Design review of the part built by this model. Coordinates are the model's own, in mm. A direction names the side the tool comes from. Give positions to 0.01 mm unless a question says otherwise; leave off trailing zeros. Loops run counter-clockwise (first coordinate to the right, second up) from the corner with the lowest first, then second, coordinate; pieces in that order, holes last. Notation, with made-up numbers: (3, 6.5) -> (53, 6.5) arc R17 ccw to (53, 36.5) -> close; hole circle Ø8 at (82, 65.5). An arc over 180 degrees is marked (long way). Answer as CSV lines item,"result".
from build123d import *

# Parameters (mm, degrees)
SKETCH1_W            = 122
SKETCH1_H            = 88
BOSS_EXTRUDE1_DEPTH  = 54
BOSS_EXTRUDE2_START  = -1
SKETCH2_W            = 118
SKETCH2_H            = 84
BOSS_EXTRUDE2_DEPTH  = 53
BOSS_EXTRUDE3_START  = 50
SKETCH3_W            = 97
SKETCH3_H            = 56
BOSS_EXTRUDE3_DEPTH  = 10
BOSS_EXTRUDE4_START  = 50
SKETCH4_R            = 4.5
BOSS_EXTRUDE4_DEPTH  = 10
BOSS_EXTRUDE5_START  = 50
SKETCH5_W            = 12
SKETCH5_H            = 6
BOSS_EXTRUDE5_DEPTH  = 10
BOSS_EXTRUDE6_START  = -65
SKETCH6_R            = 1.2
BOSS_EXTRUDE6_DEPTH  = 130
BOSS_EXTRUDE7_START  = 55
SKETCH7_R            = 1.5
BOSS_EXTRUDE7_DEPTH  = 10
BOSS_EXTRUDE8_START  = 55
SKETCH8_R            = 1.5
BOSS_EXTRUDE8_DEPTH  = 10
BOSS_EXTRUDE9_START  = 55
SKETCH9_R            = 1.5
BOSS_EXTRUDE9_DEPTH  = 10
BOSS_EXTRUDE10_START = 55
SKETCH10_R           = 1.5
BOSS_EXTRUDE10_DEPTH = 10
BOSS_EXTRUDE11_START = 55
SKETCH11_R           = 1.5
BOSS_EXTRUDE11_DEPTH = 10
BOSS_EXTRUDE12_START = 55
SKETCH12_R           = 1.5
BOSS_EXTRUDE12_DEPTH = 10
BOSS_EXTRUDE13_START = 55
SKETCH13_R           = 1.5
BOSS_EXTRUDE13_DEPTH = 10
BOSS_EXTRUDE14_START = 55
SKETCH14_R           = 1.5
BOSS_EXTRUDE14_DEPTH = 10
BOSS_EXTRUDE15_START = 55
SKETCH15_R           = 1.5
BOSS_EXTRUDE15_DEPTH = 10
BOSS_EXTRUDE16_START = 12
SKETCH16_W           = 30
SKETCH16_H           = 4
BOSS_EXTRUDE16_DEPTH = 30
BOSS_EXTRUDE17_START = -65
SKETCH17_R           = 1.1
BOSS_EXTRUDE17_DEPTH = 130
BOSS_EXTRUDE18_START = -65
SKETCH18_R           = 1.1
BOSS_EXTRUDE18_DEPTH = 130


with BuildPart() as part:
    # Sketch1 → Boss-Extrude1 (new body)
    with BuildSketch(Plane.XY):
        with Locations((0, 44)):
            Rectangle(SKETCH1_W, SKETCH1_H)
    extrude(amount=BOSS_EXTRUDE1_DEPTH)


with BuildPart() as body_2:
    # Sketch2 → Boss-Extrude2 (new body)
    with BuildSketch(Plane.XY.offset(BOSS_EXTRUDE2_START)):
        with Locations((0, 44)):
            Rectangle(SKETCH2_W, SKETCH2_H)
    extrude(amount=BOSS_EXTRUDE2_DEPTH)


with BuildPart() as part_1:
    add(part.part)

    # Combine1: cut body 2
    add(body_2.part, mode=Mode.SUBTRACT)


with BuildPart() as body_2_2:
    # Sketch3 → Boss-Extrude3 (new body)
    with BuildSketch(Plane.XY.offset(BOSS_EXTRUDE3_START)):
        with Locations((0, 42)):
            Rectangle(SKETCH3_W, SKETCH3_H)
    extrude(amount=BOSS_EXTRUDE3_DEPTH)


with BuildPart() as part_2:
    add(part_1.part)

    # Combine2: cut body 2 2
    add(body_2_2.part, mode=Mode.SUBTRACT)


with BuildPart() as body_2_3:
    # Sketch4 → Boss-Extrude4 (new body)
    with BuildSketch(Plane.XY.offset(BOSS_EXTRUDE4_START)):
        with Locations((0, 79)):
            Circle(SKETCH4_R)
    extrude(amount=BOSS_EXTRUDE4_DEPTH)


with BuildPart() as part_3:
    add(part_2.part)

    # Combine3: cut body 2 3
    add(body_2_3.part, mode=Mode.SUBTRACT)


with BuildPart() as body_2_4:
    # Sketch5 → Boss-Extrude5 (new body)
    with BuildSketch(Plane.XY.offset(BOSS_EXTRUDE5_START)):
        with Locations((34, 79)):
            Rectangle(SKETCH5_W, SKETCH5_H)
    extrude(amount=BOSS_EXTRUDE5_DEPTH)


with BuildPart() as part_4:
    add(part_3.part)

    # Combine4: cut body 2 4
    add(body_2_4.part, mode=Mode.SUBTRACT)


with BuildPart() as body_2_5:
    # Sketch6 → Boss-Extrude6 (new body)
    with BuildSketch(Plane(origin=(0, 0, 0), x_dir=(0, 0, -1), z_dir=(1, 0, 0)).offset(BOSS_EXTRUDE6_START)):
        with Locations((-27, 52)):
            Circle(SKETCH6_R)
    extrude(amount=BOSS_EXTRUDE6_DEPTH)


with BuildPart() as part_5:
    add(part_4.part)

    # Combine5: cut body 2 5
    add(body_2_5.part, mode=Mode.SUBTRACT)


with BuildPart() as body_2_6:
    # Sketch7 → Boss-Extrude7 (new body)
    with BuildSketch(Plane(origin=(0, 0, 0), x_dir=(0, 0, -1), z_dir=(1, 0, 0)).offset(BOSS_EXTRUDE7_START)):
        with Locations((-16, 20)):
            Circle(SKETCH7_R)
    extrude(amount=BOSS_EXTRUDE7_DEPTH)


with BuildPart() as part_6:
    add(part_5.part)

    # Combine6: cut body 2 6
    add(body_2_6.part, mode=Mode.SUBTRACT)


with BuildPart() as body_2_7:
    # Sketch8 → Boss-Extrude8 (new body)
    with BuildSketch(Plane(origin=(0, 0, 0), x_dir=(0, 0, -1), z_dir=(1, 0, 0)).offset(BOSS_EXTRUDE8_START)):
        with Locations((-24, 20)):
            Circle(SKETCH8_R)
    extrude(amount=BOSS_EXTRUDE8_DEPTH)


with BuildPart() as part_7:
    add(part_6.part)

    # Combine7: cut body 2 7
    add(body_2_7.part, mode=Mode.SUBTRACT)


with BuildPart() as body_2_8:
    # Sketch9 → Boss-Extrude9 (new body)
    with BuildSketch(Plane(origin=(0, 0, 0), x_dir=(0, 0, -1), z_dir=(1, 0, 0)).offset(BOSS_EXTRUDE9_START)):
        with Locations((-32, 20)):
            Circle(SKETCH9_R)
    extrude(amount=BOSS_EXTRUDE9_DEPTH)


with BuildPart() as part_8:
    add(part_7.part)

    # Combine8: cut body 2 8
    add(body_2_8.part, mode=Mode.SUBTRACT)


with BuildPart() as body_2_9:
    # Sketch10 → Boss-Extrude10 (new body)
    with BuildSketch(Plane(origin=(0, 0, 0), x_dir=(0, 0, -1), z_dir=(1, 0, 0)).offset(BOSS_EXTRUDE10_START)):
        with Locations((-16, 28)):
            Circle(SKETCH10_R)
    extrude(amount=BOSS_EXTRUDE10_DEPTH)


with BuildPart() as part_9:
    add(part_8.part)

    # Combine9: cut body 2 9
    add(body_2_9.part, mode=Mode.SUBTRACT)


with BuildPart() as body_2_10:
    # Sketch11 → Boss-Extrude11 (new body)
    with BuildSketch(Plane(origin=(0, 0, 0), x_dir=(0, 0, -1), z_dir=(1, 0, 0)).offset(BOSS_EXTRUDE11_START)):
        with Locations((-24, 28)):
            Circle(SKETCH11_R)
    extrude(amount=BOSS_EXTRUDE11_DEPTH)


with BuildPart() as part_10:
    add(part_9.part)

    # Combine10: cut body 2 10
    add(body_2_10.part, mode=Mode.SUBTRACT)


with BuildPart() as body_2_11:
    # Sketch12 → Boss-Extrude12 (new body)
    with BuildSketch(Plane(origin=(0, 0, 0), x_dir=(0, 0, -1), z_dir=(1, 0, 0)).offset(BOSS_EXTRUDE12_START)):
        with Locations((-32, 28)):
            Circle(SKETCH12_R)
    extrude(amount=BOSS_EXTRUDE12_DEPTH)


with BuildPart() as part_11:
    add(part_10.part)

    # Combine11: cut body 2 11
    add(body_2_11.part, mode=Mode.SUBTRACT)


with BuildPart() as body_2_12:
    # Sketch13 → Boss-Extrude13 (new body)
    with BuildSketch(Plane(origin=(0, 0, 0), x_dir=(0, 0, -1), z_dir=(1, 0, 0)).offset(BOSS_EXTRUDE13_START)):
        with Locations((-16, 36)):
            Circle(SKETCH13_R)
    extrude(amount=BOSS_EXTRUDE13_DEPTH)


with BuildPart() as part_12:
    add(part_11.part)

    # Combine12: cut body 2 12
    add(body_2_12.part, mode=Mode.SUBTRACT)


with BuildPart() as body_2_13:
    # Sketch14 → Boss-Extrude14 (new body)
    with BuildSketch(Plane(origin=(0, 0, 0), x_dir=(0, 0, -1), z_dir=(1, 0, 0)).offset(BOSS_EXTRUDE14_START)):
        with Locations((-24, 36)):
            Circle(SKETCH14_R)
    extrude(amount=BOSS_EXTRUDE14_DEPTH)


with BuildPart() as part_13:
    add(part_12.part)

    # Combine13: cut body 2 13
    add(body_2_13.part, mode=Mode.SUBTRACT)


with BuildPart() as body_2_14:
    # Sketch15 → Boss-Extrude15 (new body)
    with BuildSketch(Plane(origin=(0, 0, 0), x_dir=(0, 0, -1), z_dir=(1, 0, 0)).offset(BOSS_EXTRUDE15_START)):
        with Locations((-32, 36)):
            Circle(SKETCH15_R)
    extrude(amount=BOSS_EXTRUDE15_DEPTH)


with BuildPart() as part_14:
    add(part_13.part)

    # Combine14: cut body 2 14
    add(body_2_14.part, mode=Mode.SUBTRACT)


with BuildPart() as body_2_15:
    # Sketch16 → Boss-Extrude16 (new body)
    with BuildSketch(Plane.XY.offset(BOSS_EXTRUDE16_START)):
        with Locations((0, 1)):
            Rectangle(SKETCH16_W, SKETCH16_H)
    extrude(amount=BOSS_EXTRUDE16_DEPTH)


with BuildPart() as part_15:
    add(part_14.part)

    # Combine15: cut body 2 15
    add(body_2_15.part, mode=Mode.SUBTRACT)


with BuildPart() as body_2_16:
    # Sketch17 → Boss-Extrude17 (new body)
    with BuildSketch(Plane(origin=(0, 0, 0), x_dir=(0, 0, -1), z_dir=(1, 0, 0)).offset(BOSS_EXTRUDE17_START)):
        with Locations((-5, 20)):
            Circle(SKETCH17_R)
    extrude(amount=BOSS_EXTRUDE17_DEPTH)


with BuildPart() as part_16:
    add(part_15.part)

    # Combine16: cut body 2 16
    add(body_2_16.part, mode=Mode.SUBTRACT)


with BuildPart() as body_2_17:
    # Sketch18 → Boss-Extrude18 (new body)
    with BuildSketch(Plane(origin=(0, 0, 0), x_dir=(0, 0, -1), z_dir=(1, 0, 0)).offset(BOSS_EXTRUDE18_START)):
        with Locations((-5, 68)):
            Circle(SKETCH18_R)
    extrude(amount=BOSS_EXTRUDE18_DEPTH)


with BuildPart() as part_17:
    add(part_16.part)

    # Combine17: cut body 2 17
    add(body_2_17.part, mode=Mode.SUBTRACT)


solid = part_17.part
Q1. To check wall thickness, follow probe 1 along Y at (x, z) = (59.5, 32); probe 2 along Z at (x, y) = (59.95, 20); probe 3 along Z at (x, y) = (60.15, 36). State the ranges of each line that lie inside material, in increasing order. Write a range as from..to.
Filled sheet:
probe 1,"y = 0..18.5, 21.5..26.5, 29.5..34.5, 37.5..88"
probe 2,"z = 0..3.9, 6.1..14.5, 17.5..22.5, 25.5..30.5, 33.5..54"
probe 3,"z = 0..14.5, 17.5..22.5, 25.5..30.5, 33.5..54"
Q2. We need section A-A, the plane z = 32. State the section outline as (x, y) points.
Filled sheet:
outline,"(-61, 0) -> (-15, 0) -> (-15, 2) -> (-59, 2) -> (-59, 86) -> (59, 86) -> (59, 37.5) -> (61, 37.5) -> (61, 88) -> (-61, 88) -> close; (15, 0) -> (61, 0) -> (61, 18.5) -> (59, 18.5) -> (59, 2) -> (15, 2) -> close; (59, 21.5) -> (61, 21.5) -> (61, 26.5) -> (59, 26.5) -> close; (59, 29.5) -> (61, 29.5) -> (61, 34.5) -> (59, 34.5) -> close"
Q3. We need section D-D, the plane x = -32. State the section outline as (y, z) points, and give its area (3 significant figures).
Filled sheet:
outline,"(0, 0) -> (2, 0) -> (2, 52) -> (14, 52) -> (14, 54) -> (0, 54) -> close; (70, 52) -> (86, 52) -> (86, 0) -> (88, 0) -> (88, 54) -> (70, 54) -> close"
area,"272 mm^2"
Q4. We need section B-B, the plane y = 79. State the section outline as (x, z) points, and give its area (3 significant figures).
Filled sheet:
outline,"(-61, 0) -> (-59, 0) -> (-59, 52) -> (-4.5, 52) -> (-4.5, 54) -> (-61, 54) -> close; (4.5, 52) -> (28, 52) -> (28, 54) -> (4.5, 54) -> close; (40, 52) -> (59, 52) -> (59, 0) -> (61, 0) -> (61, 54) -> (40, 54) -> close"
area,"410 mm^2"
Q5. We need section C-C, the plane x = -9.5. State the section outline as (y, z) points, and give its area (3 significant figures).
Filled sheet:
outline,"(0, 0) -> (2, 0) -> (2, 12) -> (0, 12) -> close; (0, 42) -> (2, 42) -> (2, 52) -> (14, 52) -> (14, 54) -> (0, 54) -> close; (70, 52) -> (86, 52) -> (86, 0) -> (88, 0) -> (88, 54) -> (70, 54) -> close"
area,"212 mm^2"
Q6. Clearance check with flat-ended pins moving along their axes: pin 1 Ø3 at (y, z) = (52, 27) entering from +X; pin 2 Ø5.5 at (x, y) = (0, 79) entering from +Z; pin 3 Ø2 at (x, z) = (5.5, 17) entering from -Y. State where each tip first meets the part, or that it passes through.
Filled sheet:
pin 1,"stops at x = 61"
pin 2,"passes through"
pin 3,"stops at y = 86"
Q7. For faces 3 (the flat face through (-1, 88, 27)), 4 (the cylindrical face through (60, 35.1, 33.2)), 5 (the flat face through (59, 43, 26)), list the 3-axis set-ups (+Z, -Z, +X, -X, +Y, -Y) from which the entire face can be reached by the end or side of a thin tool; tool diameter is ignored.
Filled sheet:
face 3,"+Z, -Z, +X, -X, +Y"
face 4,"+X"
face 5,"-Z"
Q8. The part is to be moulded in two halves that separate along X. For faces 1 (the flat face through (-1, 86, 26)), 2 (the cylindrical face through (59.986, 29.487, 16.195)), say which applies: pulls with the +X half, pulls with the -X half, needs draft (parallel to the pull), parting line crosses it, or undercut.
Filled sheet:
face 1,"undercut"
face 2,"needs draft"
